The listing builds one solid part. Answer for the finished solid, in the listing's coordinates (mm). A direction names the side the tool comes from. Coordinates: 2 decimals unless noted, no trailing zeros. Order: outer loops, then holes, each group sorted by start corner. A loop starts at its lowest first (then second) coordinate and runs counter-clockwise, first axis right, second up. Notation, with made-up numbers: (49, -35.75) -> (106, -35.75) arc R24 cw to (106, -22.75) -> close; hole circle Ø9 at (15.5, 8). An arc over 180 degrees is marked (long way). Return JSON: item names as keys, results as strings.
Autodesk Inventor part; units mm, degrees
ref_plane "YZ Plane" through (0, 0, 0) normal (1, 0, 0) x (0, 1, 0)
ref_plane "XZ Plane" through (0, 0, 0) normal (0, 1, 0) x (-1, 0, 0)
ref_plane "XY Plane" through (0, 0, 0) normal (0, 0, 1) x (1, 0, 0)
sketch "Sketch1" plane through (-330.2, 304.8, 1412.4013) normal (0, -0.866, 0.5) x (1, 0, 0)
  line L0 (0.1333, -203.1273) -> (0, 0)
  line L1 (0, 0) -> (660.4052, 0)
  line L2 (660.4052, 0) -> (660.4052, -203.1273)
  line L3 (660.4052, -203.1273) -> (0.1333, -203.1273)
  point P0 (330.2, -1375.5753)
extrude "Extrusion1" add sketch "Sketch1" along normal blind 381
sketch "Sketch2" plane through (679.7379, 0, 139.7) normal (0, -1, 0) x (1, 0, 0)
  line L0 (-1.1909, -227.7462) -> (-1526.5875, -227.7462)
  line L1 (-1526.5875, -227.7462) -> (-1526.5875, -0.9438)
  line L2 (-1009.938, 1272.7013) -> (-1009.938, 1463.2013)
  line L3 (-1526.5875, -0.9438) -> (-1009.938, 1463.2013)
  line L4 (-349.5327, 1287.2879) -> (-349.5327, 1463.2013)
  line L5 (-1009.938, 1463.2013) -> (-349.5327, 1463.2013)
  line L6 (-349.5327, 1463.2013) -> (-1.1909, 0)
  line L7 (-1.1909, 0) -> (-1.1909, -227.7462)
  point P0 (-679.7379, -139.7)
extrude "Extrusion2" add sketch "Sketch2" along normal blind 127
sketch "Sketch3" plane through (679.7379, 0, 139.7) normal (0, 1, 0) x (1, 0, 0)
  line L0 (-1.1909, 0) -> (-349.5327, -1463.2013)
  line L1 (-346.1567, -1449.0205) -> (-1.1909, 0)
  line L2 (-1.1909, 0) -> (-123.0131, 0)
  line L3 (-349.5327, -1096.7879) -> (-349.5327, -1214.1265)
  line L4 (-123.0131, 0) -> (-349.5327, -1214.1265)
  line L5 (-349.5327, -1214.1265) -> (-349.5327, -1449.0205)
  line L6 (-349.5327, -1449.0205) -> (-346.1567, -1449.0205)
  point P0 (-679.7379, 139.7)
properties part number "esp32-s3-devkitc-1 ChipUp PinsExposed Bottom (1)"
Item 1: Which of the six approach directions +Z, -Z, +X, -X, +Y, -Y give full straight-line access (tool end or side, diameter ignored) to faces 1 (the flat face through (-73, -63, -88.046)), 2 (the flat face through (330.205, 138, 1393))?
Answer list:
{"face 1": "-Z, +X, -X, +Y, -Y", "face 2": "+Z, -Z, +X, +Y"}
Item 2: Find the intervals of material crossed by probe 1 along Y at (x, z) = (476, 868); probe 2 along X at (y, z) = (-65, 1082.5); probe 3 along Z at (x, y) = (121, 150), in increasing order.
Answer list:
{"probe 1": "-127 to 0", "probe 2": "-513.83 to 454.1", "probe 3": "1267.22 to 1501.78"}
Item 3: The part is cut by section C-C on z = 587.5. Determine the outline of the cut face in (x, y), plus the area to 3 significant figures.
Answer list:
{"outline": "(-688.5, -127) -> (571.94, -127) -> (571.94, 0) -> (-688.5, 0) -> close", "area": "160,000 mm2"}
Item 4: The part is cut by section A-A on x = -144. Determine the outline of the cut face in (y, z).
Answer list:
{"outline": "(-127, -88.05) -> (0, -88.05) -> (0, 1353.83) -> (203.24, 1236.49) -> (304.8, 1412.4) -> (0, 1588.38) -> (0, 1602.9) -> (-127, 1602.9) -> close"}
Item 5: The part is cut by section D-D on x = 421.5. Determine the outline of the cut face in (y, z), plus the area to 3 significant figures.
Answer list:
{"outline": "(-127, -88.05) -> (0, -88.05) -> (0, 1219.42) -> (-127, 1219.42) -> close", "area": "166,000 mm2"}
Item 6: Determine the mould class of faces 3 (the flat face through (4.691, 103.041, 1294.336)), 4 (the flat face through (-4.62, 154.53, 1499.16)), 5 (the flat face through (-5, -63, 1602.901)), 6 (the flat face through (-95, -127, 581)) for opening direction Y: pulls with the +Y half, pulls with the -Y half, needs draft (parallel to the pull), parting line crosses it, or undercut.
Answer list:
{"face 3": "undercut", "face 4": "pulls with the +Y half", "face 5": "needs draft", "face 6": "pulls with the -Y half"}
Item 7: Flat-ended cylindrical pins translate along their axes: pin 1 (1.5 mm diameter, centred on x = 69.5, y = 73, fed in from -Z); pin 2 (10 mm diameter, centred on x = 196.5, y = 143.5, fed in from -Z); pin 3 (12 mm diameter, centred on x = -42, y = 52, fed in from +Z). Find the tip coordinate at first contact, or state that the pin passes through.
Answer list:
{"pin 1": "z = 1311.25", "pin 2": "z = 1268.09", "pin 3": "z = 1561.82"}
Item 8: The part is cut by section B-B on y = -84.5. Determine the outline of the cut face in (x, z), plus the area to 3 significant figures.
Answer list:
{"outline": "(-846.85, -88.05) -> (678.55, -88.05) -> (678.55, 139.7) -> (330.21, 1602.9) -> (-330.2, 1602.9) -> (-846.85, 138.76) -> close", "area": "1,950,000 mm2"}
